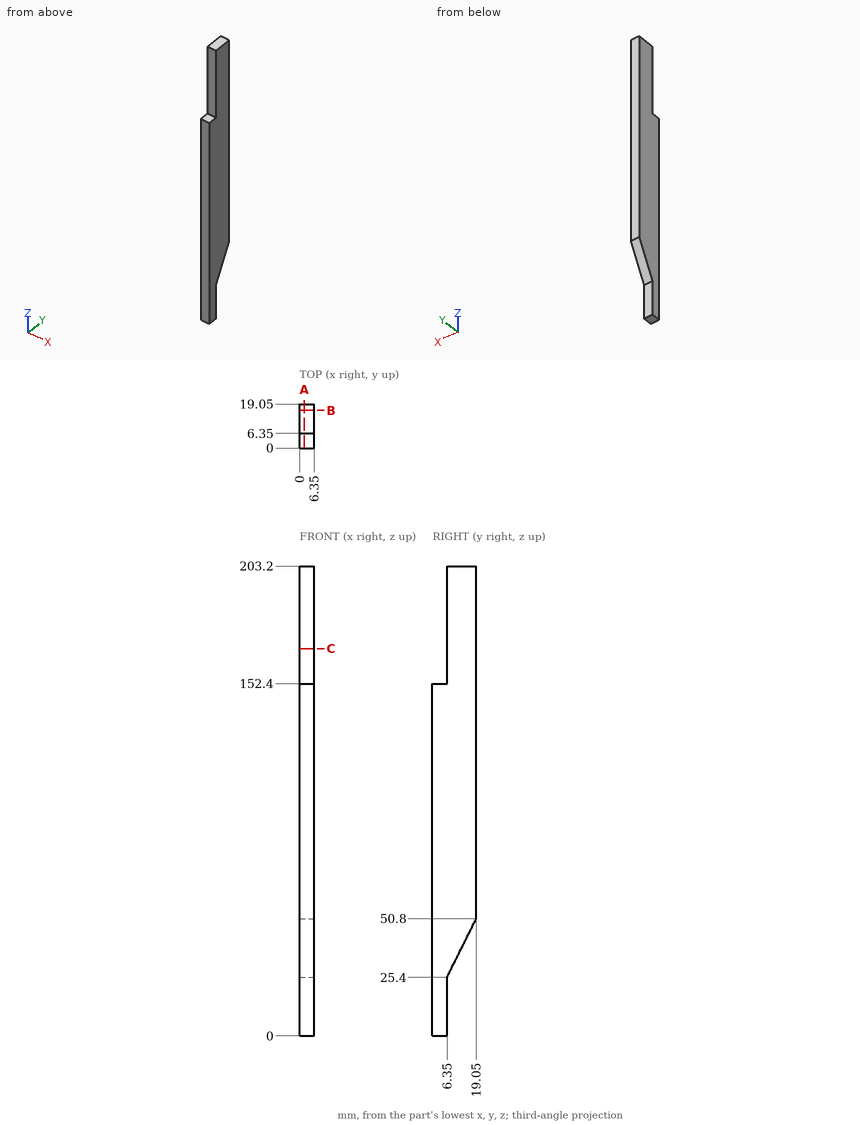
Source: three-view drawing plus pictorial views. Frame: mm from the lowest corner of the part. Coordinates: 2 decimals unless noted, no trailing zeros. Order: outer loops, then holes, each group sorted by start corner. A loop starts at its lowest first (then second) coordinate and runs counter-clockwise, first axis right, second up.
Item 1: First-contact query: P1, Ø1.5, axis at x = 3, y = 2, coming from the +Z side; P2, Ø3, axis at x = 4, z = 174, coming from the -Y side. Flat tips, straight axial feed; report the tip coordinate or a pass-through.
Output values:
P1: stops at z = 152.4
P2: stops at y = 6.35
Item 2: Material intervals for line 1 (Y direction, x = 1.5, z = 15); line 2 (Z direction, x = 2, y = 6.25); line 3 (Y direction, x = 5.5, z = 162), sorted ascending.
Output values:
line 1: y = 0 to 6.35
line 2: z = 0 to 152.4
line 3: y = 6.35 to 19.05
Item 3: Cut plane B-B (y = 16.25). Return loops of the section in (x, z), plus the area to 3 significant figures.
Output values:
outline: (0, 45.2) - (6.35, 45.2) - (6.35, 203.2) - (0, 203.2) - close
area: 1,000 mm2
Item 4: Cut plane A-A (x = 2). Return loops of the section in (y, z).
Output values:
outline: (0, 0) - (6.35, 0) - (6.35, 25.4) - (19.05, 50.8) - (19.05, 203.2) - (6.35, 203.2) - (6.35, 152.4) - (0, 152.4) - close
Item 5: Cut plane C-C (z = 167.5). Return loops of the section in (x, y), plus the area to 3 significant figures.
Output values:
outline: (0, 6.35) - (6.35, 6.35) - (6.35, 19.05) - (0, 19.05) - close
area: 80.6 mm2
